from build123d import *

# Parameters (mm, degrees)
F3_DEPTH = 1.6
F6_SIZE  = 0.2


# Not quite as in the source:
# - an extrude whose draft closes it to a point is written as a loft to that point


with BuildPart() as f1:
    # F0 (on Front) → F1 (revolve)
    with BuildSketch(Plane.XZ):
        with BuildLine():
            Line((0, 1.6), (0, -6))
            Line((0, -6), (1.5, -6))
            Line((1.5, -6), (1.5, 0))
            Line((1.5, 0), (2.75, 0))
            Line((2.75, 0), (2.75, 0.16))
            ThreePointArc((2.75, 0.16), (2.3282337649, 1.1782337649), (1.31, 1.6))
            Line((1.31, 1.6), (0, 1.6))
        make_face()
    revolve(axis=Axis((0, 0, 3.7619129732), (0, 0, 1)))

    # F2 (on face) → F3 (cut)
    with BuildSketch(Plane.XY.offset(1.6)):
        Polygon((-1, 0.5773502692), (-1, -0.5773502692), (0, -1.1547005384), (1, -0.5773502692), (1, 0.5773502692), (0, 1.1547005384), align=None)
    extrude(amount=-F3_DEPTH, mode=Mode.SUBTRACT)

    # F4 (on face) → F5 section 0
    with BuildSketch(Plane.XY, mode=Mode.PRIVATE) as f5_s0:
        Polygon((-1, 0.5773502692), (-1, -0.5773502692), (0, -1.1547005384), (1, -0.5773502692), (1, 0.5773502692), (0, 1.1547005384), align=None)
    loft([f5_s0.sketch, Vertex(0, 0, -0.3639702343)], ruled=True, mode=Mode.SUBTRACT)

    # F6
    f6_edges = [f1.edges().sort_by_distance(p)[0] for p in [
        (-1.5, 0, -6),
    ]]
    chamfer(f6_edges, length=F6_SIZE)


solid = f1.part
Design review of the part built by this model. Coordinates are the model's own, in mm. A direction names the side the tool comes from. Coordinates: 2 decimals unless noted, no trailing zeros. Write each loop counter-clockwise with the first axis right and the second up, starting at its lowest first coordinate (ties: lowest second). Pieces come first, ordered by that corner, then holes. Notation, with made-up numbers: (-14, 26) - (-5, 26) arc R14 cw to (-5, 44) - close; hole circle Ø5 at (25, -34). An arc over 180 degrees is marked (long way). One line per item, written item: value.
1) Mouldability with a two-part tool opening along Y and no side actions: class faces 1 (the face through (0, 0, -6)), 2 (the face through (-1.5, 0.07, -2.86)), 3 (the face through (-0.51, -0.86, 0.81)) as +Y half, -Y half, draft (parallel to the pull), parting line (faces both ways), or undercut.
Answer sheet:
face 1: draft
face 2: parting line
face 3: undercut
2) Insertion check: pin 1 (1 mm diameter, centred on x = 1.5, z = -4, fed in from -Y); pin 2 (0.6 mm diameter, centred on y = 0, z = 1, fed in from -X); pin 3 (1.5 mm diameter, centred on x = -2, y = -2, fed in from +Z). Each pin has a flat end and moves straight along its axis. Give the tip position at first contact, or say it passes through.
Answer sheet:
pin 1: stops at y = -1.12
pin 2: stops at x = -2.64
pin 3: stops at z = 1.38
3) To check wall thickness, follow probe 1 along Y at (x, z) = (1, -4.75); probe 2 along Z at (x, y) = (0.3, -0.3); probe 3 along X at (y, z) = (-0.7, -3.5). State the ranges of each line that lie inside material, in increasing order.
Answer sheet:
probe 1: y = -1.12 to 1.12
probe 2: z = -6 to -0.21
probe 3: x = -1.33 to 1.33
4) For faces 4 (the face through (-1.2, -1.2, 0)), 5 (the face through (-0.49, 0.87, 0.81)), list the 3-axis set-ups (+Z, -Z, +X, -X, +Y, -Y) from which the entire face can be reached by the end or side of a thin tool; tool diameter is ignored.
Answer sheet:
face 4: -Z
face 5: +Z
5) Add section A-A (z = -3.5). State the section outline as (x, y) points, plus the area to 3 significant figures.
Answer sheet:
outline: circle Ø3 at (0, 0)
area: 7.07 mm2
